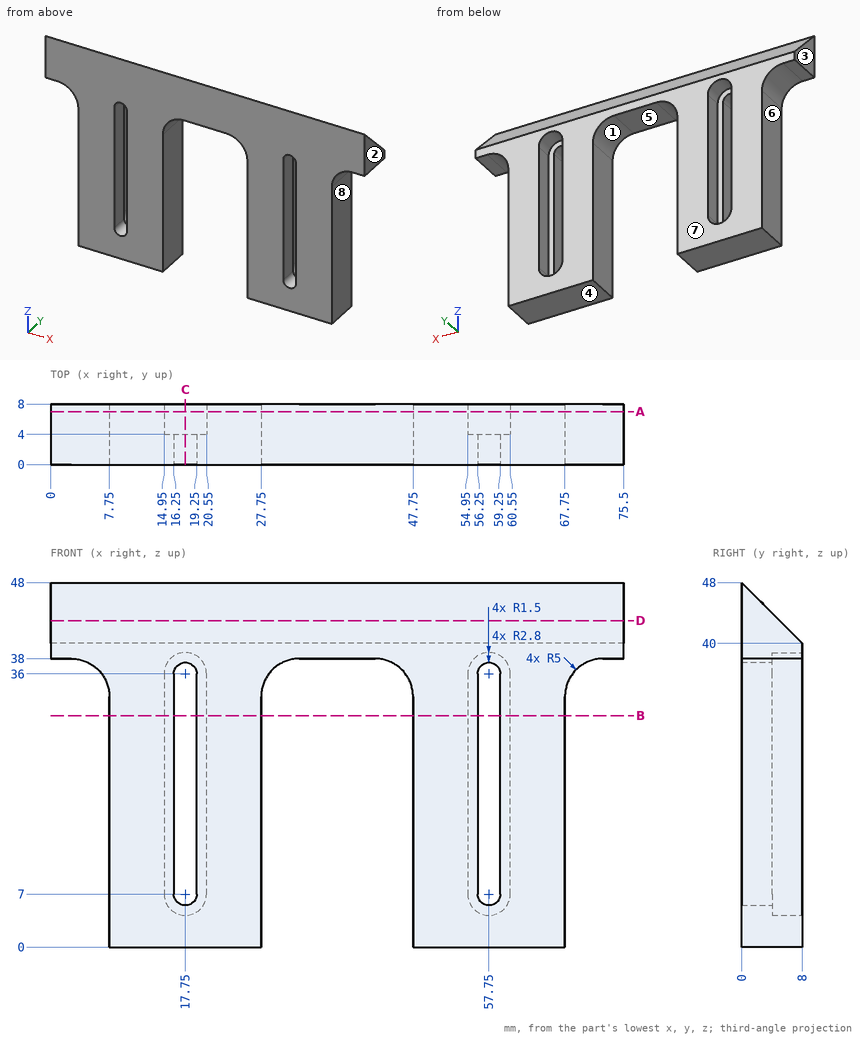
Source: three-view drawing plus pictorial views. Frame: mm from the lowest corner of the part. A direction names the side the tool comes from. Round coordinates to 2 decimals unless told otherwise and drop trailing zeros. Order: outer loops, then holes, each group sorted by start corner. A loop starts at its lowest first (then second) coordinate and runs counter-clockwise, first axis right, second up. Notation, with made-up numbers: (49, -7.5) - (108, -7.5) arc R8 cw to (108, 3.5) - close; hole circle Ø8 at (-33.75, -28.5). An arc over 180 degrees is marked (long way). Answer in a Markdown table with one row per item.
Item 1: Reachability of the marked faces 5, 6, 7 and 8 from +Z, -Z, +X, -X, +Y, -Y: full face, straight path, thin tool, end or side. Return the list, or none.
Model answer:
| item | result |
|---|---|
| face 5 | -Z, +Y, -Y |
| face 6 | -Z, -X, +Y, -Y |
| face 7 | +Z, -Z, +X, -X, +Y |
| face 8 | -Z, +X, +Y, -Y |
Item 2: Line query: line 1 (X direction, y = 1, z = 22); line 2 (X direction, y = 6, z = 31.5); line 3 (X direction, y = 7.25, z = 2.5). Output: solid intervals per line, ascending.
Model answer:
| item | result |
|---|---|
| line 1 | x = 7.75 to 16.25, 19.25 to 27.75, 47.75 to 56.25, 59.25 to 67.75 |
| line 2 | x = 7.75 to 14.95, 20.55 to 27.75, 47.75 to 54.95, 60.55 to 67.75 |
| line 3 | x = 7.75 to 27.75, 47.75 to 67.75 |
Item 3: Pin query (flat end, axial travel): pin 1 (4.5 mm diameter, centred on y = 5.5, z = 22, fed in from -X); pin 2 (2 mm diameter, centred on y = 1.5, z = 22, fed in from +X); pin 3 (1.5 mm diameter, centred on x = 36, y = 6.5, fed in from +Z); pin 4 (8 mm diameter, centred on x = 42, z = 16.5, fed in from -Y). Return the tip coordinate at first contact, or that it passes through.
Model answer:
| item | result |
|---|---|
| pin 1 | stops at x = 7.75 |
| pin 2 | stops at x = 67.75 |
| pin 3 | stops at z = 42.25 |
| pin 4 | passes through |
Item 4: Section query A-A (y = 7). Return the cut outline in (x, z), then the cut area to 3 significant figures.
Model answer:
| item | result |
|---|---|
| outline | (0, 38) - (2.75, 38) arc R5 cw to (7.75, 33) - (7.75, 0) - (27.75, 0) - (27.75, 33) arc R5 cw to (32.75, 38) - (42.75, 38) arc R5 cw to (47.75, 33) - (47.75, 0) - (67.75, 0) - (67.75, 33) arc R5 cw to (72.75, 38) - (75.5, 38) - (75.5, 41) - (0, 41) - close; hole (14.95, 7) arc R2.8 ccw to (20.55, 7) - (20.55, 36) arc R2.8 ccw to (14.95, 36) - close; hole (54.95, 7) arc R2.8 ccw to (60.55, 7) - (60.55, 36) arc R2.8 ccw to (54.95, 36) - close |
| area | 1,390 mm² |
Item 5: Section query B-B (z = 30.5). Return the cut outline in (x, y), then the cut area to 3 significant figures.
Model answer:
| item | result |
|---|---|
| outline | (7.75, 0) - (16.25, 0) - (16.25, 4) - (14.95, 4) - (14.95, 8) - (7.75, 8) - close; (19.25, 0) - (27.75, 0) - (27.75, 8) - (20.55, 8) - (20.55, 4) - (19.25, 4) - close; (47.75, 0) - (56.25, 0) - (56.25, 4) - (54.95, 4) - (54.95, 8) - (47.75, 8) - close; (59.25, 0) - (67.75, 0) - (67.75, 8) - (60.55, 8) - (60.55, 4) - (59.25, 4) - close |
| area | 251 mm² |
Item 6: Section query D-D (z = 43). Return the cut outline in (x, y), then the cut area to 4 significant figures.
Model answer:
| item | result |
|---|---|
| outline | (0, 0) - (75.5, 0) - (75.5, 5) - (0, 5) - close |
| area | 377.5 mm² |
Item 7: Mould query, pull axis X, two halves, no side actions, for the marked faces 1, 2, 3 and 4. Classes: released by +X, released by -X, zero draft, split by the parting line, or undercut.
Model answer:
| item | result |
|---|---|
| face 1 | undercut |
| face 2 | released by +X |
| face 3 | released by -X |
| face 4 | zero draft |
Item 8: Section query C-C (x = 17.75). Return the cut outline in (y, z), then the cut area to 3 significant figures.
Model answer:
| item | result |
|---|---|
| outline | (0, 0) - (8, 0) - (8, 4.2) - (4, 4.2) - (4, 5.5) - (0, 5.5) - close; (0, 37.5) - (4, 37.5) - (4, 38.8) - (8, 38.8) - (8, 40) - (0, 48) - close |
| area | 85.6 mm² |
